Source: CAD feature listing. Evaluate the final solid. Frame: model axes, mm. A direction names the side the tool comes from. Round coordinates to 2 decimals unless told otherwise and drop trailing zeros. Loops run counter-clockwise (first coordinate to the right, second up) from the corner with the lowest first, then second, coordinate; pieces in that order, holes last. Notation, with made-up numbers: M 33.25,1 L 44.25,1 A18 ccw 44.25,26 Z; hole C 37,-21 d9. An arc over 180 degrees is marked long. Answer as a JSON object with one key per item and string values.
from build123d import *

# Parameters (mm, degrees)
ESQUISSE1_R                  = 16
BOSS_EXTRU_1_DEPTH           = 38.2
ESQUISSE4_R                  = 12.5
BOSS_EXTRU_2_DEPTH           = 54.5
ESQUISSE5_R                  = 10
BOSS_EXTRU_3_DEPTH           = 3
ESQUISSE6_R                  = 3
BOSS_EXTRU_4_DEPTH           = 17
ESQUISSE8_R                  = 4
BOSS_EXTRU_5_DEPTH           = 1.2
ESQUISSE9_R                  = 3
BOSS_EXTRU_6_DEPTH           = 1.5
ESQUISSE10_R                 = 1.5
BOSS_EXTRU_7_DEPTH           = 13
ESQUISSE11_W                 = 0.4
ESQUISSE11_H                 = 2.4
BOSS_EXTRU_8_DEPTH           = 8.3
ESQUISSE14_R                 = 0.9
ENL_V_MAT_EXTRU_2_DEPTH      = 1
R_P_TITION_CIRCULAIRE3_COUNT = 2
R_P_TITION_CIRCULAIRE4_COUNT = 2
ESQUISSE15_R                 = 0.8
ENL_V_MAT_EXTRU_3_DEPTH      = 3
R_P_TITION_CIRCULAIRE5_COUNT = 2
ESQUISSE16_R                 = 1.5
ENL_V_MAT_EXTRU_4_DEPTH      = 4
R_P_TITION_CIRCULAIRE6_COUNT = 4


with BuildPart() as part:
    # Esquisse1 → Boss.-Extru.1 (new body)
    with BuildSketch(Plane.XY):
        Circle(ESQUISSE1_R)
    extrude(amount=BOSS_EXTRU_1_DEPTH)

    # Esquisse4 → Boss.-Extru.2 (add)
    with BuildSketch(Plane(origin=(0, 0, 0), x_dir=(-1, 0, 0), z_dir=(0, 0, -1))):
        with Locations(Location((0, 0, 0), (0, 0, 180))):
            Circle(ESQUISSE4_R)
    extrude(amount=BOSS_EXTRU_2_DEPTH)

    # Esquisse5 → Boss.-Extru.3 (add)
    with BuildSketch(Plane.XY.offset(38.2)):
        Circle(ESQUISSE5_R)
    extrude(amount=BOSS_EXTRU_3_DEPTH)

    # Esquisse6 → Boss.-Extru.4 (add)
    with BuildSketch(Plane.XY.offset(41.2)):
        Circle(ESQUISSE6_R)
    extrude(amount=BOSS_EXTRU_4_DEPTH)

    # Esquisse8 → Boss.-Extru.5 (add)
    with BuildSketch(Plane(origin=(0, 0, -54.5), x_dir=(-1, 0, 0), z_dir=(0, 0, -1))):
        Circle(ESQUISSE8_R)
    extrude(amount=BOSS_EXTRU_5_DEPTH)

    # Esquisse9 → Boss.-Extru.6 (add)
    with BuildSketch(Plane(origin=(0, 0, -55.7), x_dir=(-1, 0, 0), z_dir=(0, 0, -1))):
        with Locations(Location((0, 0, 0), (0, 0, 180))):
            Circle(ESQUISSE9_R)
    extrude(amount=BOSS_EXTRU_6_DEPTH)

    # Esquisse10 → Boss.-Extru.7 (add)
    with BuildSketch(Plane(origin=(0, 0, -57.2), x_dir=(-1, 0, 0), z_dir=(0, 0, -1))):
        with Locations(Location((0, 0, 0), (0, 0, 180))):
            Circle(ESQUISSE10_R)
    extrude(amount=BOSS_EXTRU_7_DEPTH)

    # Esquisse11 → Boss.-Extru.8 (add)
    with BuildSketch(Plane(origin=(0, 0, -54.5), x_dir=(-1, 0, 0), z_dir=(0, 0, -1))):
        with Locations((-8.8, 0.9)):
            Rectangle(ESQUISSE11_W, ESQUISSE11_H)
    boss_extru_8 = extrude(amount=BOSS_EXTRU_8_DEPTH)

    # Esquisse14 → Enlèv. mat.-Extru.2 (cut)
    with BuildSketch(Plane(origin=(9, 0, 0), x_dir=(0, 0, -1), z_dir=(1, 0, 0))):
        with Locations((59.997923429, 0.92616233)):
            Circle(ESQUISSE14_R)
    enl_v_mat_extru_2 = extrude(amount=-ENL_V_MAT_EXTRU_2_DEPTH, mode=Mode.SUBTRACT)

    # Répétition circulaire3: Boss.-Extru.8 ×2 about axis
    r_p_tition_circulaire3_axis = Axis((0, 0, 0), (0, 0, 1))
    for i in range(1, R_P_TITION_CIRCULAIRE3_COUNT):
        add(boss_extru_8.rotate(r_p_tition_circulaire3_axis, i * 360 / R_P_TITION_CIRCULAIRE3_COUNT))

    # Répétition circulaire4: Enlèv. mat.-Extru.2 ×2 about axis
    r_p_tition_circulaire4_axis = Axis((0, 0, -70.2), (0, 0, 1))
    for i in range(1, R_P_TITION_CIRCULAIRE4_COUNT):
        add(enl_v_mat_extru_2.rotate(r_p_tition_circulaire4_axis, i * 360 / R_P_TITION_CIRCULAIRE4_COUNT), mode=Mode.SUBTRACT)

    # Esquisse15 → Enlèv. mat.-Extru.3 (cut)
    with BuildSketch(Plane(origin=(0, 0, -54.5), x_dir=(-1, 0, 0), z_dir=(0, 0, -1))):
        with Locations((-4.210841648, 7.596559423)):
            Circle(ESQUISSE15_R)
    enl_v_mat_extru_3 = extrude(amount=-ENL_V_MAT_EXTRU_3_DEPTH, mode=Mode.SUBTRACT)

    # Répétition circulaire5: Enlèv. mat.-Extru.3 ×2 about axis
    r_p_tition_circulaire5_axis = Axis((0, 0, 0), (0, 0, 1))
    for i in range(1, R_P_TITION_CIRCULAIRE5_COUNT):
        add(enl_v_mat_extru_3.rotate(r_p_tition_circulaire5_axis, i * 360 / R_P_TITION_CIRCULAIRE5_COUNT), mode=Mode.SUBTRACT)

    # Esquisse16 → Enlèv. mat.-Extru.4 (cut)
    with BuildSketch(Plane.XY.offset(38.2)):
        with Locations((-13, 0)):
            Circle(ESQUISSE16_R)
    enl_v_mat_extru_4 = extrude(amount=-ENL_V_MAT_EXTRU_4_DEPTH, mode=Mode.SUBTRACT)

    # Répétition circulaire6: Enlèv. mat.-Extru.4 ×4 about axis
    r_p_tition_circulaire6_axis = Axis((0, 0, 0), (0, 0, 1))
    for i in range(1, R_P_TITION_CIRCULAIRE6_COUNT):
        add(enl_v_mat_extru_4.rotate(r_p_tition_circulaire6_axis, i * 360 / R_P_TITION_CIRCULAIRE6_COUNT), mode=Mode.SUBTRACT)


solid = part.part
Item 1: Line query: probe 1 along Z at (x, y) = (13, 5.5); probe 2 along Z at (x, y) = (-1.5, -8); probe 3 along Y at (x, z) = (-13, 36). Output: solid intervals per line, ascending. Write a range as from..to.
Answer sheet:
{"probe 1": "z = 0..38.2", "probe 2": "z = -54.5..41.2", "probe 3": "y = -9.33..-1.5, 1.5..9.33"}
Item 2: Pull-direction query (Y, two-part tool) for faces 1 (the cylindrical face through (-0.07, -14.5, 36.23)), 2 (the cylindrical face through (0.07, 14.5, 36.23)), 3 (the cylindrical face through (1.43, -0.45, -63.61)), 4 (the flat face through (-0.2, -10.4, 38.2)); classes: pulls with the +Y half, pulls with the -Y half, needs draft (parallel to the pull), parting line crosses it, or undercut.
Answer sheet:
{"face 1": "undercut", "face 2": "undercut", "face 3": "parting line crosses it", "face 4": "needs draft"}
Item 3: Section A-A on z = 49.5. Return the cut outline in (x, y).
Answer sheet:
{"outline": "C 0,0 d6"}
Item 4: Access query for faces 5 (the cylindrical face through (-14.5, 0.07, 36.23)), 6 (the cylindrical face through (0.867, -3.905, -55.092)), 7 (the flat face through (9, 0.9, -58.6)), 8 (the flat face through (0, 0, 58.2)). Directions: +Z, -Z, +X, -X, +Y, -Y. A direction counts if a zero-diameter tool reaches every point of the face in a straight line with its end or side. Return the directions, or none.
Answer sheet:
{"face 5": "+Z", "face 6": "-Z", "face 7": "-Z, +X, +Y, -Y", "face 8": "+Z, +X, -X, +Y, -Y"}
Item 5: Section C-C on z = -29.5. Return the cut outline in (x, y).
Answer sheet:
{"outline": "C 0,0 d25"}
Item 6: Section B-B on x = 6.5. Return the cut outline in (y, z).
Answer sheet:
{"outline": "M -14.62,0 L -10.68,0 L -10.68,-54.5 L 10.68,-54.5 L 10.68,0 L 14.62,0 L 14.62,38.2 L 7.6,38.2 L 7.6,41.2 L -7.6,41.2 L -7.6,38.2 L -14.62,38.2 Z"}
Item 7: Contact query for flat-ended pins moving along their axis: pin 1 Ø0.7 at (y, z) = (-0.5, -58.5) entering from +X; pin 2 Ø8 at (y, z) = (8, 28.5) entering from -X; pin 3 Ø2 at (y, z) = (-9.5, -30) entering from +X; pin 4 Ø16 at (x, y) = (3.5, 5.5) entering from -Z. Output: stop coordinate, or through.
Answer sheet:
{"pin 1": "stops at x = 9", "pin 2": "stops at x = -15.49", "pin 3": "stops at x = 9.17", "pin 4": "stops at z = -70.2"}
